Autodesk Inventor part; units mm, degrees
ref_plane "YZ Plane" through (0, 0, 0) normal (1, 0, 0) x (0, 1, 0)
ref_plane "XZ Plane" through (0, 0, 0) normal (0, 1, 0) x (-1, 0, 0)
ref_plane "XY Plane" through (0, 0, 0) normal (0, 0, 1) x (1, 0, 0)
ref_plane "РабПлоскость1" through (0, 0, 0) normal (0, 0, 1) x (1, 0, 0)
sketch "Эскиз1" plane through (0, 0, 0) normal (0, 0, 1) x (1, 0, 0)
  circle A0 centre (0, 75) radius 8
  circle A1 centre (0, -75) radius 8
  line L0 (34.641, -80) -> (60.6218, -35)
  arc A2 (60.6218, -35) -> (60.6218, 35) centre (0, 0) ccw
  line L1 (60.6218, 35) -> (34.641, 80)
  arc A3 (34.641, 80) -> (-34.641, 80) centre (0, 60) ccw
  line L2 (-34.641, 80) -> (-60.6218, 35)
  arc A4 (-60.6218, 35) -> (-60.6218, -35) centre (0, 0) ccw
  line L3 (-60.6218, -35) -> (-34.641, -80)
  arc A5 (-34.641, -80) -> (34.641, -80) centre (0, -60) ccw
  circle A6 centre (0, 0) radius 50
  circle A7 centre (0, 75) radius 11
  circle A8 centre (0, -75) radius 11
  point P0 (0, 0)
  dimension "d22" = 22
  dimension "d23" = 22
extrude "Выдавливание1" add sketch "Эскиз1" along normal blind 50 contours A5 L3 A4 L2 A3 L1 A2 L0 | A6
sketch "Эскиз2" plane through (0, 0, 0) normal (0, 0, -1) x (-1, 0, 0)
  circle A0 centre (0, 0) radius 50
  dimension "d2" = 100
extrude "Выдавливание2" add sketch "Эскиз2" along normal blind 15
sketch "Эскиз3" plane through (0, 0, 50) normal (0, 0, 1) x (1, 0, 0)
  circle A0 centre (0, 0) radius 45
  dimension "d5" = 90
extrude "Выдавливание3" add sketch "Эскиз3" along normal blind 25
fillet "Сопряжение1" radius 10 1 edges at (-45, 0, 50)
sketch "Эскиз4" plane through (0, 0, 75) normal (0, 0, 1) x (1, 0, 0)
  circle A0 centre (0, 0) radius 55
  circle A1 centre (0, 0) radius 22.5
  dimension "d9" = 45
extrude "Выдавливание4" cut sketch "Эскиз4" against normal through all contours A1
chamfer "Фаска1" distance 2 angle 45 3 edges at (-22.5, 0, 75) (50, 0, -15) (-22.5, 0, -15)
sketch "Эскиз5" plane through (0, 0, 0) normal (1, 0, 0) x (0, 1, 0)
  line L0 (-24.5, -15) -> (24.5, -15)
  line L1 (48, -15) -> (-48, -15)
  line L2 (22.5, 73) -> (22.5, -13)
  line L3 (22.5, -15) -> (22.5, -8)
  line L4 (22.5, -8) -> (27.5, -8)
  line L5 (27.5, -8) -> (29.3756, -15)
  line L6 (0, -32.6) -> (0, 90.6)
  point P0 (0, 0)
  dimension "d15" = 7
  dimension "d16" = 5
  dimension "d17" = 105
revolve "Вращение1" cut sketch "Эскиз5" angle 360 about axis through (0, 0, -10) along (0, 0, 1)
chamfer "Фаска2" distance 2 angle 45 1 edges at (-22.5, 0, -8)
properties part number "Фланецгайка" material "Сталь, углеродистая"
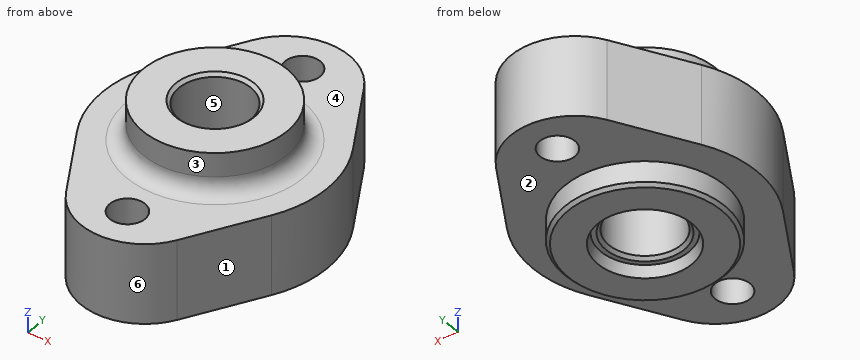
Input: part model. Units: mm. Frame: model coordinates. Face numbers are marked on the shaded views. A direction names the side the tool comes from. Give positions to 0.01 mm unless a question says otherwise; leave off trailing zeros. Write each loop counter-clockwise with the first axis right and the second up, starting at its lowest first coordinate (ties: lowest second). Pieces come first, ordered by that corner, then holes. Notation, with made-up numbers: M 19.25,37 L 31.25,37 A30 ccw 31.25,64 Z; hole C 29,72.5 d10. An arc over 180 degrees is marked long. Use one line per item in the form item = value.
1. Cut plane A-A on y = 0. Return loops of the section in (x, z).
Outcome:
outline = M -70,0 L -50,0 L -50,-13 L -48,-15 L -29.38,-15 L -27.5,-8 L -24.5,-8 L -22.5,-6 L -22.5,73 L -24.5,75 L -45,75 L -45,60 A10 cw -55,50 L -70,50 Z; M 22.5,-6 L 24.5,-8 L 27.5,-8 L 29.38,-15 L 48,-15 L 50,-13 L 50,0 L 70,0 L 70,50 L 55,50 A10 cw 45,60 L 45,75 L 24.5,75 L 22.5,73 Z
2. Mould query, pull axis Y, two halves, no side actions, for the marked faces 4, 5 and 6. Classes: released by +Y, released by -Y, zero draft, split by the parting line, or undercut.
Outcome:
face_4 = zero draft
face_5 = undercut
face_6 = released by -Y
3. Cut plane C-C on x = 0. State how many separate pieces and enclosed holes the cut face has, and give its area (3 significant figures).
Outcome:
separate_pieces = 4
enclosed_holes = 0
area = 7,450 mm²
4. First-contact query: P1, Ø4, axis at x = -13, z = 16.5, coming from the -Y side; P2, Ø10, axis at y = -78, z = 53, coming from the -X side; P3, Ø8, axis at y = 72.5, z = 7.5, coming from the +X side. Flat tips, straight axial feed; report the tip coordinate or a pass-through.
Outcome:
P1 = -98.46
P2 = -38.11
P3 = 41.28
5. Cut plane B-B on z = 11. Return loops of the section in (x, y).
Outcome:
outline = M -60.62,-35 L -34.64,-80 A40 ccw 34.64,-80 L 60.62,-35 A70 ccw 60.62,35 L 34.64,80 A40 ccw -34.64,80 L -60.62,35 A70 ccw Z; hole C 0,0 d45; hole C 0,-75 d22; hole C 0,75 d22
6. Ray query, L1, parallel to X at y = 0, z = 13; L2, parallel to Y at x = 9.5, z = 3; L3, parallel to Z at x = -28.5, y = -88. Return the intervals inside material, ascending.
Outcome:
L1 = -70 to -22.5, 22.5 to 70
L2 = -98.86 to -80.55, -69.45 to -20.4, 20.4 to 69.45, 80.55 to 98.86
L3 = 0 to 50
7. Reachability of the marked faces 1, 2 and 3 from +Z, -Z, +X, -X, +Y, -Y: full face, straight path, thin tool, end or side. Return the list, or none.
Outcome:
face_1 = +Z, -Z, +X, -Y
face_2 = -Z
face_3 = +Z
8. Cut plane D-D on z = 63. Return loops of the section in (x, y).
Outcome:
outline = C 0,0 d90; hole C 0,0 d45
